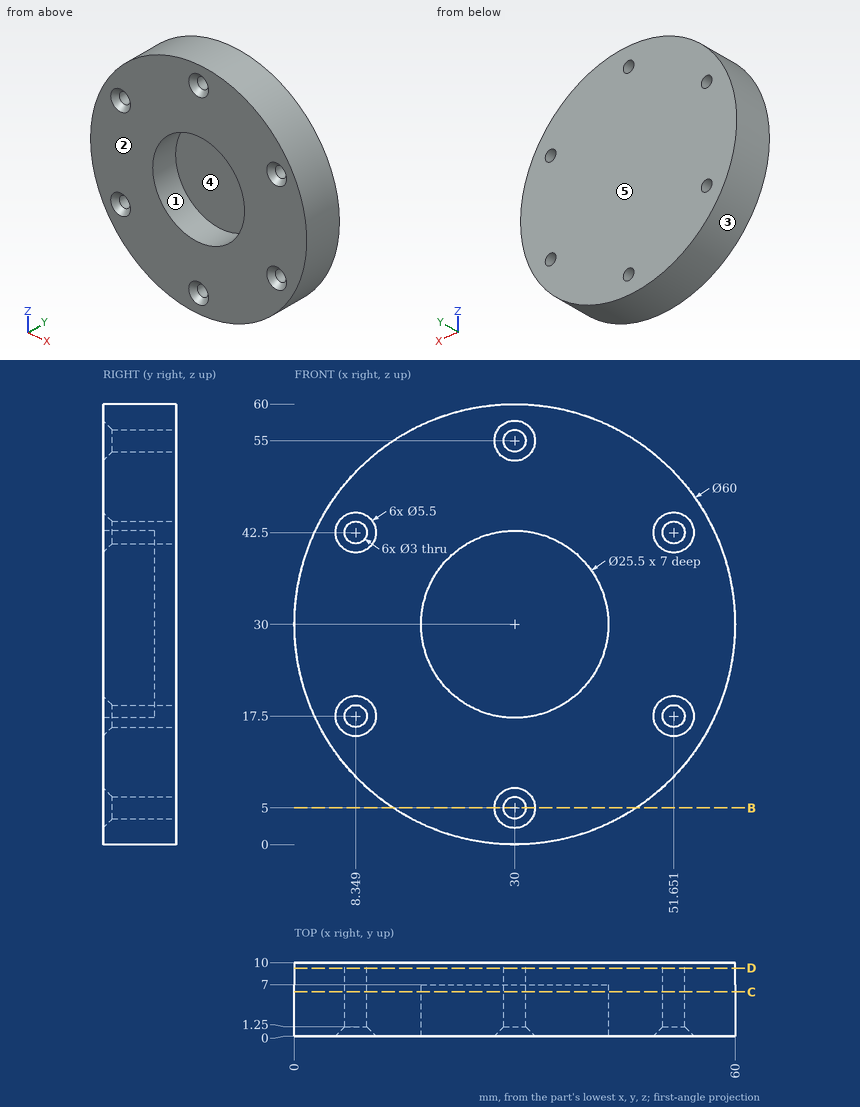
Job drawing, mm, ordinate dimensions from the low corner. One solid piece. A direction names the side the tool comes from. Give positions to 0.01 mm unless a question says otherwise; leave off trailing zeros. Write each loop counter-clockwise with the first axis right and the second up, starting at its lowest first coordinate (ties: lowest second). Pieces come first, ordered by that corner, then holes. Notation, with made-up numbers: M 15.5,77.25 L 38.5,77.25 A16 cw 38.5,91.25 Z; hole C 51,-37.5 d8. An arc over 180 degrees is marked long. One line per item, written item: value. Start each with the question number.
Q1. Drop flat-ended pins along their axis: pin 1 Ø4 at (y, z) = (4.5, 23) entering from -X; pin 2 Ø3.5 at (x, z) = (8.35, 42.5) entering from -Y; pin 3 Ø5 at (x, y) = (10, 7.5) entering from -Z. Give the stop position or say it passes through.
Q2. Saw through at D-D, the plane y = 9.25. Write the cut outline in (x, z), plus the area to 4 significant figures.
Q3. Probe probe 1 along Z at (x, y) = (30, 5.75); probe 2 along Z at (x, y) = (25, 1.25); probe 3 along Z at (x, y) = (37.5, 2). List the from-to ranges inside material, lowest first. Write a range as [from, to].
Q4. 3-axis set-ups, long thin cutter, end or side, ignore diameter. For the marked faces 1 and 2: which of +Z, -Z, +X, -X, +Y, -Y reach the whole face in a straight line?
Q5. Two-plate mould, pull along Z, no slides. Class the marked faces 3, 4 and 5: +Z half, -Z half, draft (parallel to the pull), parting line (faces both ways), or undercut.
Q6. Saw through at B-B, the plane z = 5. Write the cut outline in (x, y).
Q7. Saw through at C-C, the plane y = 6. Write the cut outline in (x, z), plus the area to 3 significant figures.
Output values:
1. pin 1: stops at x = 0.42
1. pin 2: stops at y = 1
1. pin 3: stops at z = 5.63
2. outline: C 30,30 d60; hole C 8.35,17.5 d3; hole C 8.35,42.5 d3; hole C 30,5 d3; hole C 30,55 d3; hole C 51.65,17.5 d3; hole C 51.65,42.5 d3
2. area: 2,785 mm²
3. probe 1: z = [0, 3.5], [6.5, 17.25], [42.75, 53.5], [56.5, 60]
3. probe 2: z = [0.42, 18.27], [41.73, 59.58]
3. probe 3: z = [0.95, 19.69], [40.31, 59.05]
4. face 1: -Y
4. face 2: +Z, -Z, +X, -X, -Y
5. face 3: parting line
5. face 4: undercut
5. face 5: draft
6. outline: M 13.42,0 L 27.25,0 L 28.5,1.25 L 28.5,10 L 13.42,10 Z; M 31.5,1.25 L 32.75,0 L 46.58,0 L 46.58,10 L 31.5,10 Z
7. outline: C 30,30 d60; hole C 8.35,17.5 d3; hole C 8.35,42.5 d3; hole C 30,30 d25.5; hole C 30,5 d3; hole C 30,55 d3; hole C 51.65,17.5 d3; hole C 51.65,42.5 d3
7. area: 2,270 mm²
